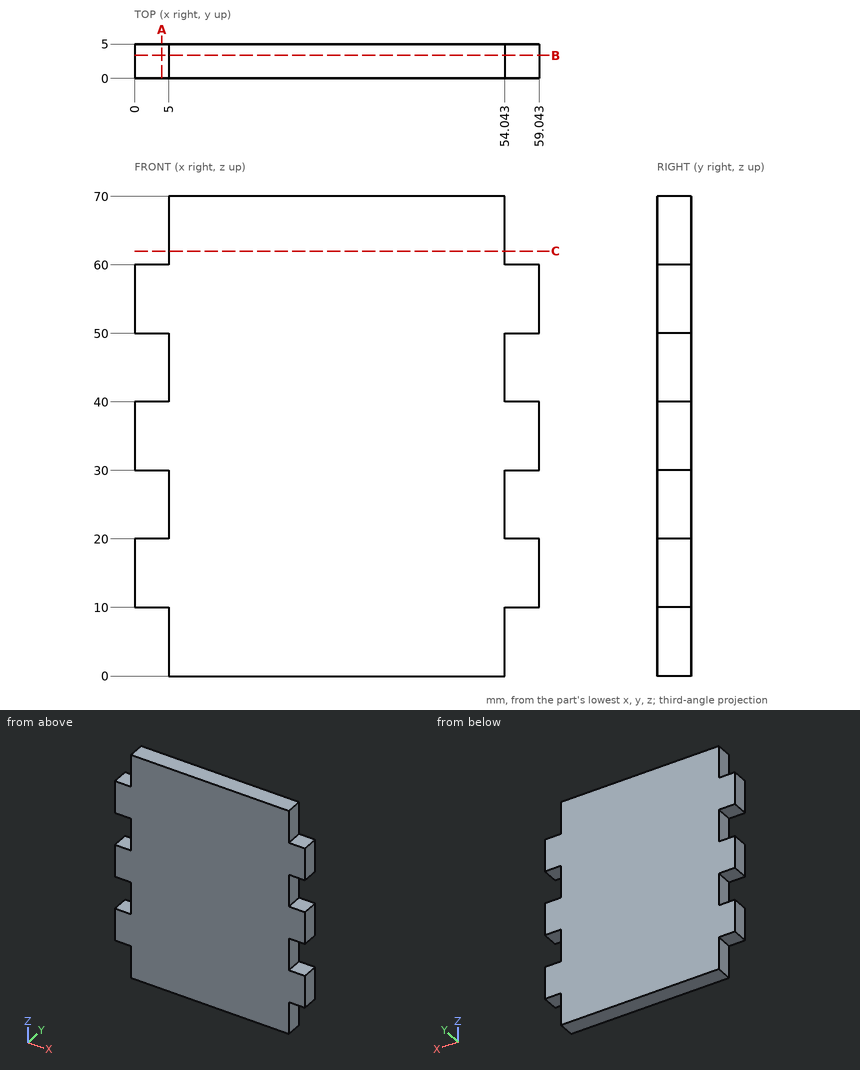
Geometry: see drawing. Coordinates: mm, zero at the bounding-box minimum. Give positions to 0.01 mm unless a question says otherwise; leave off trailing zeros. Loops run counter-clockwise (first coordinate to the right, second up) from the corner with the lowest first, then second, coordinate; pieces in that order, holes last. Notation, with made-up numbers: (7.25, -31) -> (52.25, -31) arc R23 cw to (52.25, -5) -> close; hole circle Ø3 at (3.25, -21.5). An arc over 180 degrees is marked (long way). Put each result on its own line as item: value.
1. Cut plane C-C (z = 62). Return the cut outline in (x, y), plus the area to 3 significant figures.
Taken from the geometry:
outline: (5, 0) -> (54.04, 0) -> (54.04, 5) -> (5, 5) -> close
area: 245 mm2
2. Ray query, line 1 along Z through (x, y) = (3, 2.4); line 2 along X through (y, z) = (2.55, 27). Return the intervals inside material, ascending. Write a range as [from, to].
Taken from the geometry:
line 1: z = [10, 20], [30, 40], [50, 60]
line 2: x = [5, 54.04]
3. Pin query (flat end, axial travel): P1, Ø1.5, axis at x = 3, y = 3.5, coming from the +Z side; P2, Ø8, axis at x = 29, z = 8.5, coming from the -Y side; P3, Ø2.5, axis at y = 3.5, z = 66, coming from the -X side; P4, Ø1.5, axis at y = 3.5, z = 3, coming from the +X side. Return the tip coordinate at first contact, or that it passes through.
Taken from the geometry:
P1: stops at z = 60
P2: stops at y = 0
P3: stops at x = 5
P4: stops at x = 54.04
4. Cut plane B-B (y = 3.35). Return the cut outline in (x, z), plus the area to 3 significant figures.
Taken from the geometry:
outline: (0, 10) -> (5, 10) -> (5, 0) -> (54.04, 0) -> (54.04, 10) -> (59.04, 10) -> (59.04, 20) -> (54.04, 20) -> (54.04, 30) -> (59.04, 30) -> (59.04, 40) -> (54.04, 40) -> (54.04, 50) -> (59.04, 50) -> (59.04, 60) -> (54.04, 60) -> (54.04, 70) -> (5, 70) -> (5, 60) -> (0, 60) -> (0, 50) -> (5, 50) -> (5, 40) -> (0, 40) -> (0, 30) -> (5, 30) -> (5, 20) -> (0, 20) -> close
area: 3,730 mm2
5. Cut plane A-A (x = 4). Return the cut outline in (y, z).
Taken from the geometry:
outline: (0, 10) -> (5, 10) -> (5, 20) -> (0, 20) -> close; (0, 30) -> (5, 30) -> (5, 40) -> (0, 40) -> close; (0, 50) -> (5, 50) -> (5, 60) -> (0, 60) -> close
